Can you work these out from the model? Positions are in its coordinate system, mm. Face numbers are marked on the shaded views. A direction names the side the tool comes from. Give positions to 0.01 mm unless a question says otherwise; leave off trailing zeros. Loops run counter-clockwise (first coordinate to the right, second up) from the corner with the lowest first, then second, coordinate; pieces in that order, holes last. Notation, with made-up numbers: (-22.75, 51.5) - (-8.75, 51.5) arc R10 cw to (-8.75, 55.5) - close; hole circle Ø4 at (73, 12.25). An arc over 180 degrees is marked (long way). Use a Markdown table: item, result. Add a question column.
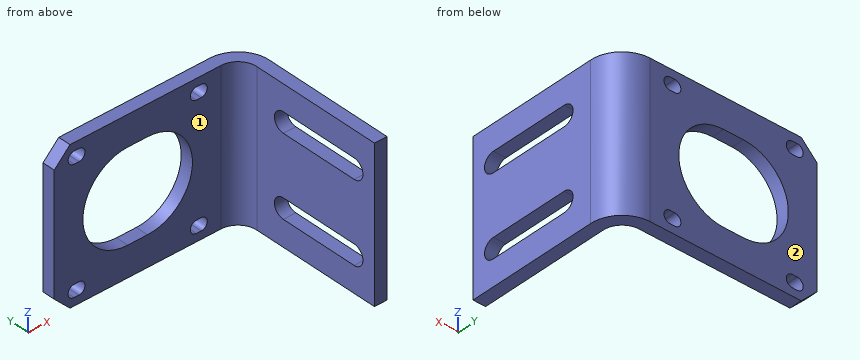
```python
from build123d import *

# Parameters (mm, degrees)
SKETCH1_W                    = 38
SKETCH1_H                    = 38
BASE_FLANGE1_DEPTH           = 3.175
EDGE_FLANGE1_STRIP_W         = 22.225
EDGE_FLANGE1_STRIP_H         = 3.175
EDGE_FLANGE1_STRIP_CUT_DEPTH = 38
EDGE_FLANGE1_DEPTH           = 38
EDGE_FLANGE1_START           = 3.175
EDGE_FLANGE1_PROFILE_W       = 38
EDGE_FLANGE1_PROFILE_H       = 42.3
EDGE_FLANGE1_FLAT_DEPTH      = 3.175
CHAMFER1_SIZE                = 4
CUT_EXTRUDE1_DEPTH           = 10


# Sheet-metal steps are written as plain solids
with BuildPart() as part:
    # Sketch1 → Base-Flange1 (new body)
    with BuildSketch(Plane.ZY.offset(-22.559027455)):
        with Locations((229.809714632, 54.911820509)):
            Rectangle(SKETCH1_W, SKETCH1_H)
    extrude(amount=BASE_FLANGE1_DEPTH)

    # Edge-Flange1 strip (across the edge) → Edge-Flange1 strip cut (cut)
    with BuildSketch(Plane(origin=(19.384027455, 73.911820509, 248.809714632), x_dir=(0, -1, 0), z_dir=(0, 0, -1))):
        with Locations((-6.35, -1.5875)):
            Rectangle(EDGE_FLANGE1_STRIP_W, EDGE_FLANGE1_STRIP_H)
    extrude(amount=EDGE_FLANGE1_STRIP_CUT_DEPTH, mode=Mode.SUBTRACT)

    # Edge-Flange1 bend section (across the edge) → Edge-Flange1 (add)
    with BuildSketch(Plane(origin=(19.384027455, 73.911820509, 248.809714632), x_dir=(0, -1, 0), z_dir=(0, 0, -1))):
        with BuildLine():
            Line((-3.175, 4.7625), (0, 4.7625))
            ThreePointArc((0, 4.7625), (1.394903955, 1.394903955), (4.7625, 0))
            Line((4.7625, 0), (4.7625, -3.175))
            ThreePointArc((4.7625, -3.175), (-0.850160076, -0.850160076), (-3.175, 4.7625))
        make_face()
    extrude(amount=EDGE_FLANGE1_DEPTH)

    # Edge-Flange1 profile (on flange) → Edge-Flange1 flat (add)
    with BuildSketch(Plane(origin=(19.384027455, 73.911820509, 0), x_dir=(0, 0, -1), z_dir=(0, 1, 0)).offset(EDGE_FLANGE1_START)):
        with Locations((-229.809714632, 25.9125)):
            Rectangle(EDGE_FLANGE1_PROFILE_W, EDGE_FLANGE1_PROFILE_H)
        with BuildLine():
            Line((-246.850058636, 9.810559352), (-246.850058636, 11.014440648))
            ThreePointArc((-246.850058636, 11.014440648), (-245.309714632, 12.554784652), (-243.769370628, 11.014440648))
            Line((-243.769370628, 11.014440648), (-243.769370628, 9.810559352))
            ThreePointArc((-243.769370628, 9.810559352), (-245.309714632, 8.270215348), (-246.850058636, 9.810559352))
        make_face(mode=Mode.SUBTRACT)
        with BuildLine():
            Line((-215.850058636, 9.810559352), (-215.850058636, 11.014440648))
            ThreePointArc((-215.850058636, 11.014440648), (-214.309714632, 12.554784652), (-212.769370628, 11.014440648))
            Line((-212.769370628, 11.014440648), (-212.769370628, 9.810559352))
            ThreePointArc((-212.769370628, 9.810559352), (-214.309714632, 8.270215348), (-215.850058636, 9.810559352))
        make_face(mode=Mode.SUBTRACT)
        with BuildLine():
            Line((-241.197832947, 23.4125), (-241.197832947, 28.4125))
            ThreePointArc((-241.197832947, 28.4125), (-229.809714632, 39.800618315), (-218.421596317, 28.4125))
            Line((-218.421596317, 28.4125), (-218.421596317, 23.4125))
            ThreePointArc((-218.421596317, 23.4125), (-229.809714632, 12.024381685), (-241.197832947, 23.4125))
        make_face(mode=Mode.SUBTRACT)
        with BuildLine():
            Line((-246.850058636, 40.810559352), (-246.850058636, 42.014440648))
            ThreePointArc((-246.850058636, 42.014440648), (-245.309714632, 43.554784652), (-243.769370628, 42.014440648))
            Line((-243.769370628, 42.014440648), (-243.769370628, 40.810559352))
            ThreePointArc((-243.769370628, 40.810559352), (-245.309714632, 39.270215348), (-246.850058636, 40.810559352))
        make_face(mode=Mode.SUBTRACT)
        with BuildLine():
            Line((-215.850058636, 40.810559352), (-215.850058636, 42.014440648))
            ThreePointArc((-215.850058636, 42.014440648), (-214.309714632, 43.554784652), (-212.769370628, 42.014440648))
            Line((-212.769370628, 42.014440648), (-212.769370628, 40.810559352))
            ThreePointArc((-212.769370628, 40.810559352), (-214.309714632, 39.270215348), (-215.850058636, 40.810559352))
        make_face(mode=Mode.SUBTRACT)
    extrude(amount=-EDGE_FLANGE1_FLAT_DEPTH)

    # Chamfer1
    chamfer1_edges = [part.edges().sort_by_distance(p)[0] for p in [
        (-27.678472545, 75.499320509, 248.809714632),
        (-27.678472545, 75.499320509, 210.809714632),
    ]]
    chamfer(chamfer1_edges, length=CHAMFER1_SIZE)

    # Sketch9 → Cut-Extrude1 (cut)
    with BuildSketch(Plane.ZY.offset(-19.384027455)):
        with BuildLine():
            Line((242.309714632, 61.660898278), (242.309714632, 41.660898278))
            ThreePointArc((242.309714632, 41.660898278), (239.809714632, 39.160898278), (237.309714632, 41.660898278))
            Line((237.309714632, 41.660898278), (237.309714632, 61.660898278))
            ThreePointArc((237.309714632, 61.660898278), (239.809714632, 64.160898278), (242.309714632, 61.660898278))
        make_face()
        with BuildLine():
            Line((222.309714633, 61.660898278), (222.309714633, 41.660898278))
            ThreePointArc((222.309714633, 41.660898278), (219.809714633, 39.160898278), (217.309714633, 41.660898278))
            Line((217.309714633, 41.660898278), (217.309714633, 61.660898278))
            ThreePointArc((217.309714633, 61.660898278), (219.809714633, 64.160898278), (222.309714633, 61.660898278))
        make_face()
    extrude(amount=-CUT_EXTRUDE1_DEPTH, mode=Mode.SUBTRACT)


solid = part.part
```
1. Please list where these lines run through material, in increasing order: line 1 along X through (y, z) = (49.5, 216); line 2 along Y through (x, z) = (-17, 238); line 3 along Z through (x, y) = (-15, 74.5). Write a range as [from, to].
2. Suppose I cut it at C-C (z = 226.5). List the corners of the cut face in (x, y) for me (1 decimal), and give its area (3 significant figures).
3. Suppose I cut it at A-A (y = 43.5). List the corners of the cut face in (x, z) for me.
4. Suppose I cut it at D-D (z = 238). List the corners of the cut face in (x, y) for me (1 decimal).
5. Will these pins go through, and if not, where does the flat tip stop? P1, Ø1.5, axis at y = 69.5, z = 233.5, coming from the -X side; P2, Ø1.5, axis at y = 66.5, z = 238, coming from the -X side; P3, Ø1.5, axis at x = 5.5, z = 220.5, coming from the -Y side; P4, Ø8, axis at x = 2.5, y = 69.5, coming from the -Z side.
6. On a 3-axis mill with a long thin cutter (end or side, diameter ignored), from which of +Z, -Z, +X, -X, +Y, -Y can I reach the whole of each face in a straight line? I mean the marked faces 1 and 2. Say none if no direction works.
7. Suppose I cut it at B-B (x = -6). List the corners of the cut face in (y, z) for me, and give its area (3 significant figures).
Results below:
| question | item | result |
|---|---|---|
| 1 | line 1 | [19.38, 22.56] |
| 1 | line 2 | [73.91, 77.09] |
| 1 | line 3 | [210.81, 220.11], [239.51, 248.81] |
| 2 | outline | (-27.7, 73.9) - (-19.9, 73.9) - (-19.9, 77.1) - (-27.7, 77.1) - close; (6.9, 73.9) - (14.6, 73.9) arc R4.8 cw to (19.4, 69.1) - (19.4, 35.9) - (22.6, 35.9) - (22.6, 69.1) arc R7.9 ccw to (14.6, 77.1) - (6.9, 77.1) - close |
| 2 | area | 186 mm² |
| 3 | outline | (19.38, 210.81) - (22.56, 210.81) - (22.56, 217.31) - (19.38, 217.31) - close; (19.38, 222.31) - (22.56, 222.31) - (22.56, 237.31) - (19.38, 237.31) - close; (19.38, 242.31) - (22.56, 242.31) - (22.56, 248.81) - (19.38, 248.81) - close |
| 4 | outline | (-27.7, 73.9) - (-16.9, 73.9) - (-16.9, 77.1) - (-27.7, 77.1) - close; (3.9, 73.9) - (14.6, 73.9) arc R4.8 cw to (19.4, 69.1) - (19.4, 63.4) - (22.6, 63.4) - (22.6, 69.1) arc R7.9 ccw to (14.6, 77.1) - (3.9, 77.1) - close; (19.4, 35.9) - (22.6, 35.9) - (22.6, 39.9) - (19.4, 39.9) - close |
| 5 | P1 | x = 19.26 |
| 5 | P2 | x = 19.38 |
| 5 | P3 | y = 73.91 |
| 5 | P4 | through |
| 6 | face 1 | +Z, -Z, -X, -Y |
| 6 | face 2 | +Z, -Z, +X, -X, +Y |
| 7 | outline | (73.91, 210.81) - (77.09, 210.81) - (77.09, 218.42) - (73.91, 218.42) - close; (73.91, 241.2) - (77.09, 241.2) - (77.09, 248.81) - (73.91, 248.81) - close |
| 7 | area | 48.3 mm² |
